Input: dimensioned drawing with shaded views. Units: mm. Origin: part minimum x, y, z. A direction names the side the tool comes from. Give positions to 0.01 mm unless a question says otherwise; leave off trailing zeros. Loops run counter-clockwise (first coordinate to the right, second up) from the corner with the lowest first, then second, coordinate; pieces in that order, holes last. Notation, with made-up numbers: (22, 77.25) -> (73, 77.25) arc R20 cw to (73, 107.25) -> close; hole circle Ø1 at (39.25, 45). An arc over 180 degrees is marked (long way). Answer as a JSON object with one key per item and string values.
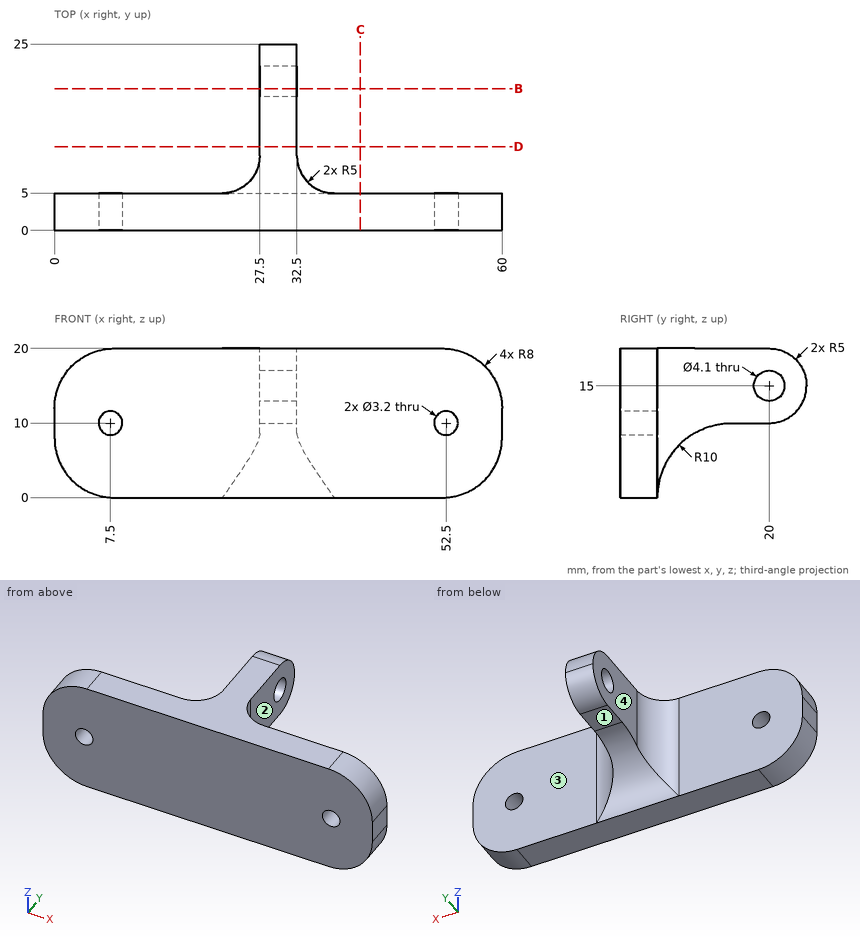
Q1. Pin query (flat end, axial travel): pin 1 (5.5 mm diameter, centred on y = 16, z = 16.5, fed in from +X); pin 2 (4 mm diameter, centred on x = 16.5, z = 16, fed in from +Y); pin 3 (3.5 mm diameter, centred on y = 20, z = 15, fed in from +X); pin 4 (4 mm diameter, centred on x = 29, y = 18.5, fed in from -Z). Return the tip coordinate at first contact, or that it passes through.
Evaluation:
{"pin 1": "stops at x = 32.5", "pin 2": "stops at y = 5", "pin 3": "passes through", "pin 4": "stops at z = 10"}
Q2. Ray query, line 1 along X through (y, z) = (2.55, 10); line 2 along Y through (x, z) = (29.1, 15); line 3 along Y through (x, z) = (56.5, 16.75). Return the intervals inside material, ascending.
Evaluation:
{"line 1": "x = 0 to 5.9, 9.1 to 50.9, 54.1 to 60", "line 2": "y = 0 to 17.95, 22.05 to 25", "line 3": "y = 0 to 5"}
Q3. Section B-B, the plane y = 19. Return the cut outline in (x, z).
Evaluation:
{"outline": "(27.5, 10) -> (32.5, 10) -> (32.5, 13.21) -> (27.5, 13.21) -> close; (27.5, 16.79) -> (32.5, 16.79) -> (32.5, 20) -> (27.5, 20) -> close"}
Q4. Access query for the marked faces 1, 2, 3 and 4. Directions: +Z, -Z, +X, -X, +Y, -Y. A direction counts if a zero-diameter tool reaches every point of the face in a straight line with its end or side. Return the directions, or none.
Evaluation:
{"face 1": "-Z, +X, -X, +Y", "face 2": "+Z, -Z, +X, +Y", "face 3": "+Z, -Z, +X, +Y", "face 4": "+Z, -Z, -X, +Y"}
Q5. Section C-C, the plane x = 41. Return the cut outline in (y, z).
Evaluation:
{"outline": "(0, 0) -> (5, 0) -> (5, 20) -> (0, 20) -> close"}
Q6. Section D-D, the plane y = 11.25. Return the cut outline in (x, z).
Evaluation:
{"outline": "(27.5, 9.27) -> (32.5, 9.27) -> (32.5, 20) -> (27.5, 20) -> close"}
